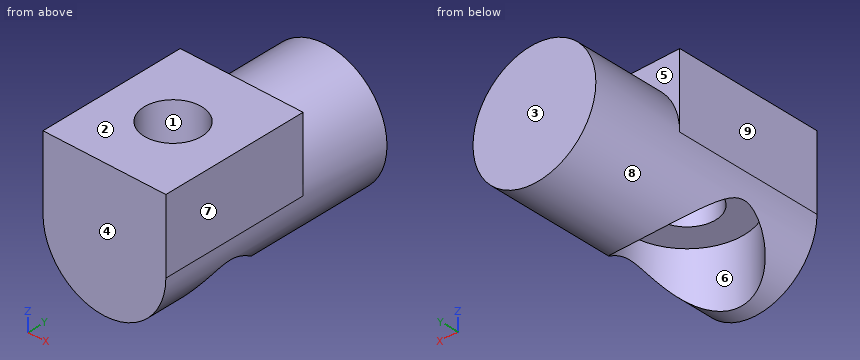
Solid Edge part; units mm, degrees
sketch "Sketch1" plane through (0, 0, 0) normal (0, -1, 0) x (1, 0, 0)
  circle A0 centre (0, 0) radius 3.75
extrude "Protrusion1" add sketch "Sketch1" along normal blind 14.5
sketch "Sketch2" plane through (0, -14.5, 0) normal (0, -1, 0) x (1, 0, 0)
  line L0 (-3.75, 4.5) -> (3.75, 4.5)
  line L1 (3.75, 0) -> (3.75, 4.5)
  line L2 (-3.75, 0) -> (3.75, 0)
  line L3 (-3.75, 0) -> (-3.75, 4.5)
extrude "ExtrudedCutout_1" add sketch "Sketch2" against normal blind 9
sketch "Sketch3" plane through (0, 0, 0) normal (0, 0, -1) x (-1, 0, 0)
  circle A0 centre (0, -10) radius 3.5
extrude "ExtrudedCutout_4" cut sketch "Sketch3" along normal blind 4
sketch "Sketch4" plane through (0, 0, 0) normal (0, 0, -1) x (-1, 0, 0)
  circle A0 centre (0, -10) radius 1.75
extrude "Cutout1" cut sketch "Sketch4" against normal up to vertex (4.5 mm away)
properties material "Polycarbonate"
Verification items for the finished model (mm, model axes). Face numbers are marked on the shaded views. A direction names the side the tool comes from. Coordinates: 2 decimals unless noted, no trailing zeros. Order: outer loops, then holes, each group sorted by start corner. A loop starts at its lowest first (then second) coordinate and runs counter-clockwise, first axis right, second up. Notation, with made-up numbers: M 63.25,65 L 112.25,65 A10 cw 112.25,76 Z; hole C 8,30.25 d8. An arc over 180 degrees is marked long. One line per item, written item: value. Start each with the question number.
Item 1: Sectioned sample at B-B on y = -11.25. Record the cut outline in (x, z), then the cut area to 3 significant figures.
Item 2: Depth check by flat-ended pin: P1, Ø3, axis at x = -0.5, z = -1, coming from the +Y side; P2, Ø3.5, axis at x = -1.5, y = -10.5, coming from the -Z side. Enter the tip coordinate at first touch or a pass-through.
Item 3: Sectioned sample at C-C on z = 4.25. Record the cut outline in (x, y), then the cut area to 3 significant figures.
Item 4: Mould release check, pull along Y, two halves, no side actions. Record for the marked faces 1, 2, 3 and 4: pulls with the +Y half, pulls with the -Y half, needs draft (parallel to the pull), parting line crosses it, or undercut.
Item 5: Sectioned sample at D-D on y = -9.25. Record the cut outline in (x, z).
Item 6: Sectioned sample at A-A on x = 0. Record the cut outline in (y, z).
Item 7: Thickness scan on probe 1 along Y at (x, z) = (0, 3.55); probe 2 along Y at (x, z) = (0, -2.65); probe 3 along Z at (x, y) = (1.25, -12.5). Record the ranges inside material, lowest first.
Item 8: Access from +Z, -Z, +X, -X, +Y, -Y to the whole of each face (thin tool, end or side, straight path). Record for the marked faces 5, 6, 7, 8 and 9.
Calculated:
1. outline: M -3.75,0 A3.75 ccw -3.27,-1.84 L -3.27,0 L -1.22,0 L -1.22,4.5 L -3.75,4.5 Z; M 1.22,0 L 3.27,0 L 3.27,-1.84 A3.75 ccw 3.75,0 L 3.75,4.5 L 1.22,4.5 Z
1. area: 23.9 mm^2
2. P1: y = 0
2. P2: z = 0
3. outline: M -3.75,-14.5 L 3.75,-14.5 L 3.75,-5.5 L -3.75,-5.5 Z; hole C 0,-10 d3.5
3. area: 57.9 mm^2
4. face 1: undercut
4. face 2: needs draft
4. face 3: pulls with the +Y half
4. face 4: pulls with the -Y half
5. outline: M -3.75,0 A3.75 ccw -3.42,-1.54 L -3.42,0 L -1.58,0 L -1.58,4.5 L -3.75,4.5 Z; M 1.58,0 L 3.42,0 L 3.42,-1.54 A3.75 ccw 3.75,0 L 3.75,4.5 L 1.58,4.5 Z
6. outline: M -14.5,-3.75 L -13.5,-3.75 L -13.5,0 L -11.75,0 L -11.75,4.5 L -14.5,4.5 Z; M -8.25,0 L -6.5,0 L -6.5,-3.75 L 0,-3.75 L 0,3.75 L -5.5,3.75 L -5.5,4.5 L -8.25,4.5 Z
7. probe 1: -14.5 to -11.75, -8.25 to 0
7. probe 2: -14.5 to -13.5, -6.5 to 0
7. probe 3: 0 to 4.5
8. face 5: +Z, +Y
8. face 6: -Z
8. face 7: +Z, -Z, +X, +Y, -Y
8. face 8: +Y
8. face 9: +Z, -Z, -X, +Y, -Y
